from build123d import *

# Parameters (mm, degrees)
F0_W      = 5
F0_H      = 20
F1_DEPTH  = 5
F2_R      = 3
F3_DEPTH  = 5
F4_R      = 3
F5_DEPTH  = 5
F6_R      = 1.35
F7_DEPTH  = 5
F8_R      = 1.45
F9_DEPTH  = 5
F10_W     = 5
F10_H     = 10
F11_DEPTH = 5


with BuildPart() as f1:
    # F0 (on Top) → F1 (new body)
    with BuildSketch(Plane.XY):
        Rectangle(F0_W, F0_H)
    extrude(amount=F1_DEPTH)

    # F2 (on Top) → F3 (join)
    with BuildSketch(Plane.XY):
        with Locations((0, 10)):
            Circle(F2_R)
    extrude(amount=F3_DEPTH)

    # F4 (on Top) → F5 (join)
    with BuildSketch(Plane.XY):
        with Locations((0, -10)):
            Circle(F4_R)
    extrude(amount=F5_DEPTH)

    # F6 (on face) → F7 (cut)
    with BuildSketch(Plane.XY.offset(5)):
        with Locations((0, 10)):
            Circle(F6_R)
    extrude(amount=-F7_DEPTH, mode=Mode.SUBTRACT)

    # F8 (on face) → F9 (cut)
    with BuildSketch(Plane.XY.offset(5)):
        with Locations((0, -10)):
            Circle(F8_R)
    extrude(amount=-F9_DEPTH, mode=Mode.SUBTRACT)

    # F10 (on face) → F11 (join)
    with BuildSketch(Plane.XY.offset(5)):
        Rectangle(F10_W, F10_H)
    extrude(amount=F11_DEPTH)


solid = f1.part
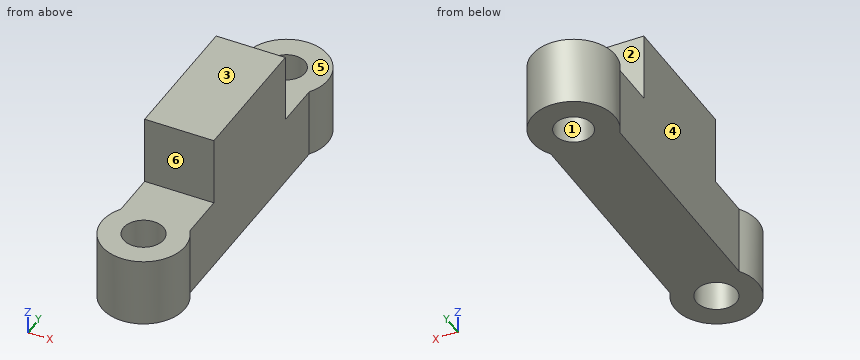
CAD build for the part. Positions are in the model's coordinates, mm. Face numbers are marked on the shaded views. A direction names the side the tool comes from. Coordinates: 2 decimals unless noted, no trailing zeros. Write each loop counter-clockwise with the first axis right and the second up, starting at its lowest first coordinate (ties: lowest second). Pieces come first, ordered by that corner, then holes. Notation, with made-up numbers: M 4.5,-22.5 L 23.5,-22.5 A19 cw 23.5,-1.5 Z; hole C 21,12.5 d3. An arc over 180 degrees is marked long. Return JSON: item names as keys, results as strings.
Item 1: Slice it at B-B, the plane x = 0.6. Write the cut outline in (y, z).
Findings below:
{"outline": "M -12.94,0 L -11.32,0 L -11.32,5 L -12.94,5 Z; M -8.68,0 L 8.79,0 L 8.79,5 L 5,5 L 5,10 L -5,10 L -5,5 L -8.68,5 Z; M 11.21,0 L 12.94,0 L 12.94,5 L 11.21,5 Z"}
Item 2: Two-plate mould, pull along Y, no slides. Class the marked faces 1, 2 and 3: +Y half, -Y half, draft (parallel to the pull), parting line (faces both ways), or undercut.
Findings below:
{"face 1": "undercut", "face 2": "+Y half", "face 3": "draft"}
Item 3: Slice it at C-C, the plane z = 2.5. Write the cut outline in (x, y).
Findings below:
{"outline": "M -2.5,-8.34 A3 ccw long 2.5,-8.34 L 2.5,8.34 A3 ccw long -2.5,8.34 Z; hole C 0,-10 d2.9; hole C 0,10 d2.7"}
Item 4: Probe line 1 (Y direction, x = 0, z = 1.3); line 2 (Y direction, x = -0.9, z = 4.5); line 3 (X direction, y = -7, z = 4). List the from-to ranges inside material, lowest first. Write a range as from..to.
Findings below:
{"line 1": "y = -13..-11.45, -8.55..8.65, 11.35..13", "line 2": "y = -12.86..-11.14, -8.86..8.99, 11.01..12.86", "line 3": "x = -2.5..2.5"}
Item 5: Slice it at A-A, the plane y = -10. Write the cut outline in (x, z), and give its area (3 significant figures).
Findings below:
{"outline": "M -3,0 L -1.45,0 L -1.45,5 L -3,5 Z; M 1.45,0 L 3,0 L 3,5 L 1.45,5 Z", "area": "15.5 mm2"}
Item 6: Drop flat-ended pins along their axis: pin 1 Ø3 at (y, z) = (1, 3.5) entering from -X; pin 2 Ø3 at (x, y) = (-1.5, -9.5) entering from +Z; pin 3 Ø1 at (y, z) = (9, 1.5) entering from -X. Give the stop position or say it passes through.
Findings below:
{"pin 1": "stops at x = -2.5", "pin 2": "stops at z = 5", "pin 3": "stops at x = -2.96"}
Item 7: Slice it at D-D, the plane y = 10. Write the cut outline in (x, z).
Findings below:
{"outline": "M -3,0 L -1.35,0 L -1.35,5 L -3,5 Z; M 1.35,0 L 3,0 L 3,5 L 1.35,5 Z"}
Item 8: Which spindle directions (+Z, -Z, +X, -X, +Y, -Y) get a long thin tool onto all of the face, cutting with end or side? Do the marked faces 4, 5 and 6. Say none if no direction does.
Findings below:
{"face 4": "+Z, -Z, -X", "face 5": "+Z, +X, -X, +Y", "face 6": "+Z, +X, -X, -Y"}
